Source: CAD feature listing. Evaluate the final solid. Frame: model axes, mm. A direction names the side the tool comes from. Give positions to 0.01 mm unless a question says otherwise; leave off trailing zeros. Write each loop counter-clockwise with the first axis right and the second up, starting at its lowest first coordinate (ties: lowest second). Pieces come first, ordered by that corner, then holes.
```python
from build123d import *

# Parameters (mm, degrees)
SKETCH1_R           = 12.7
BOSS_EXTRUDE1_DEPTH = 177.8
BOSS_EXTRUDE2_DEPTH = 25.4


with BuildPart() as part:
    # Sketch1 → Boss-Extrude1 (new body)
    with BuildSketch(Plane(origin=(0, 0, 0), x_dir=(1, 0, 0), z_dir=(0, 1, 0))):
        Circle(SKETCH1_R)
    boss_extrude1 = extrude(amount=BOSS_EXTRUDE1_DEPTH)

    # Sketch2 → Boss-Extrude2 (add)
    with BuildSketch(Plane(origin=(0, 177.8, 0), x_dir=(1, 0, 0), z_dir=(0, 1, 0))):
        with BuildLine():
            Line((-12.7, 0), (-12.7, 203.2))
            Line((-12.7, 203.2), (12.7, 203.2))
            Line((12.7, 203.2), (12.7, 0))
            ThreePointArc((12.7, 0), (0, -12.7), (-12.7, 0))
        make_face()
    boss_extrude2 = extrude(amount=BOSS_EXTRUDE2_DEPTH)

    # Mirror1: Boss-Extrude1, Boss-Extrude2 across plane
    add(boss_extrude1.mirror(Plane(origin=(0, 0, 0), x_dir=(0, 0, 1), z_dir=(0, -1, 0))))
    add(boss_extrude2.mirror(Plane(origin=(0, 0, 0), x_dir=(0, 0, 1), z_dir=(0, -1, 0))))


solid = part.part
```
1. Mould query, pull axis Y, two halves, no side actions, for faces 1 (the flat face through (0, -190, -203.2)), 2 (the flat face through (0, -177.8, -103)), 3 (the flat face through (0, 203.2, -97)). Classes: +Y half, -Y half, draft (parallel to the pull), parting line (faces both ways), or undercut.
2. Contact query for a flat-ended pin moving along its axis: P1, Ø6, axis at x = 3, y = -61, coming from the -Z side. Output: stop coordinate, or through.
3. Access query for faces 4 (the flat face through (-12.7, 190, -100)), 5 (the cylindrical face through (-1.653, 2.845, 12.592)). Directions: +Z, -Z, +X, -X, +Y, -Y. A direction counts if a zero-diameter tool reaches every point of the face in a straight line with its end or side. Return the directions, or none.
4. Cut plane B-B, the plane x = 0. Return the cut outline in (y, z).
5. Cut plane C-C, the plane y = 68.5. Return the cut outline in (x, z), then the cut area to 3 significant figures.
6. Cut plane A-A, the plane z = -188. Return the cut outline in (x, y), then the cut area to 3 significant figures.
7. Line query: L1, parallel to Y at x = -11.25, z = -157.5; L2, parallel to Z at x = 0.25, y = -6.5; L3, parallel to X at y = -151, z = 2.5. Output: solid intervals per line, ascending.
Response values:
1. face 1: draft
1. face 2: undercut
1. face 3: +Y half
2. P1: stops at z = -12.7
3. face 4: +Z, -Z, -X, +Y, -Y
3. face 5: none
4. outline: (-203.2, -203.2) - (-177.8, -203.2) - (-177.8, -12.7) - (177.8, -12.7) - (177.8, -203.2) - (203.2, -203.2) - (203.2, 12.7) - (-203.2, 12.7) - close
5. outline: circle Ø25.4 at (0, 0)
5. area: 507 mm2
6. outline: (-12.7, -203.2) - (12.7, -203.2) - (12.7, -177.8) - (-12.7, -177.8) - close; (-12.7, 177.8) - (12.7, 177.8) - (12.7, 203.2) - (-12.7, 203.2) - close
6. area: 1,290 mm2
7. L1: y = -203.2 to -177.8, 177.8 to 203.2
7. L2: z = -12.7 to 12.7
7. L3: x = -12.45 to 12.45
